Design review of the part built by this model. Coordinates are the model's own, in mm. A direction names the side the tool comes from. Round coordinates to 2 decimals unless told otherwise and drop trailing zeros. Order: outer loops, then holes, each group sorted by start corner. A loop starts at its lowest first (then second) coordinate and runs counter-clockwise, first axis right, second up. Notation, with made-up numbers: (70, -25.75) - (116, -25.75) arc R21 cw to (116, 13.25) - close; hole circle Ø6 at (-10, -35.75). An arc over 180 degrees is marked (long way). Write item = value, one per line.
from build123d import *

# Parameters (mm, degrees)
SKETCH_1_R          = 5
SKETCH_1_R_2        = 2.5
EXTRUDE_1_DEPTH     = 10
EXTRUDE_1_2_DEPTH   = 10
EXTRUDE_2_DEPTH     = 6
CUT_EXTRUDE_1_DEPTH = 4
SKETCH_5_R          = 2.5
EXTRUDE_3_DEPTH     = 2
CUT_EXTRUDE_2_DEPTH = 4


with BuildPart() as part:
    # Sketch 1 → Extrude 1 (new body)
    with BuildSketch(Plane.XY):
        with Locations((-11.277859903, 1.201925786)):
            Circle(SKETCH_1_R)
        with Locations((-11.277859903, 1.201925786)):
            Circle(SKETCH_1_R_2, mode=Mode.SUBTRACT)
    extrude(amount=EXTRUDE_1_DEPTH)



with BuildPart() as body_2:
    # Sketch 1 → Extrude 1 2 (new body)
    with BuildSketch(Plane.XY):
        with Locations((-37.440810807, -24.961025118)):
            Circle(SKETCH_1_R)
        with Locations((-37.440810807, -24.961025118)):
            Circle(SKETCH_1_R_2, mode=Mode.SUBTRACT)
    extrude(amount=EXTRUDE_1_2_DEPTH)


with BuildPart() as part_1:
    add(part.part)

    add(body_2.part)  # Extrude 2 merges body 2
    # Sketch 3 → Extrude 2 (add)
    with BuildSketch(Plane(origin=(0, 0, 0), x_dir=(-1, 0, 0), z_dir=(0, 0, -1))):
        Polygon((11.277859903, 1.201925786), (14.813393809, 4.737459692), (40.976344713, -21.425491212), (33.905276901, -28.496559024), (7.742325997, -2.33360812), align=None)
    extrude(amount=-EXTRUDE_2_DEPTH)

    # Sketch 4 → Cut-Extrude 1 (cut)
    with BuildSketch(Plane.XY.offset(6)):
        Polygon((-13.045626856, 2.969692739), (-9.51009295, -0.565841167), (-35.673043854, -26.728792071), (-39.20857776, -23.193258165), align=None)
    extrude(amount=-CUT_EXTRUDE_1_DEPTH, mode=Mode.SUBTRACT)

    # Sketch 5 → Extrude 3 (add)
    with BuildSketch(Plane(origin=(0, 0, 0), x_dir=(-1, 0, 0), z_dir=(0, 0, -1))):
        with Locations(Location((11.277859903, 1.201925786, 0), (0, 0, 45))):
            Circle(SKETCH_5_R)
        with Locations(Location((37.440810807, -24.961025118, 0), (0, 0, 45))):
            Circle(SKETCH_5_R)
    extrude(amount=-EXTRUDE_3_DEPTH)

    # Sketch 4_2 → Cut-Extrude 2 (cut)
    with BuildSketch(Plane.XY.offset(6)):
        Polygon((-13.045626856, 2.969692739), (-9.51009295, -0.565841167), (-35.673043854, -26.728792071), (-39.20857776, -23.193258165), align=None)
    extrude(amount=CUT_EXTRUDE_2_DEPTH, mode=Mode.SUBTRACT)


solid = part_1.part
1) The part is to be moulded in two halves that separate along X. For faces 3 (the flat face through (-21.01, -15.6, 2.96)), 4 (the flat face through (-24, -12, 2)), 5 (the cylindrical face through (-41.104, -28.365, 6.041)), 6 (the flat face through (-27, -9, 6)), say which applies: released by +X, released by -X, zero draft, split by the parting line, or undercut.
Findings:
face_3 = released by +X
face_4 = undercut
face_5 = split by the parting line
face_6 = zero draft
2) We need section B-B on y = -26. Write out the cut boundary in (x, z).
Findings:
outline = (-42.33, 0) - (-31.41, 0) - (-31.41, 6) - (-32.55, 6) - (-32.55, 10) - (-34.94, 10) - (-34.94, 2) - (-39.71, 2) - (-39.71, 10) - (-42.33, 10) - close
3) We need section D-D on z = 8. Write out the cut boundary in (x, y), and give its area (3 significant figures).
Findings:
outline = (-39.21, -23.19) - (-36.15, -20.13) arc R5 ccw (long way) to (-32.61, -23.67) - (-35.67, -26.73) arc R2.5 cw to start; (-16.11, -0.09) - (-13.05, 2.97) arc R2.5 cw to (-9.51, -0.57) - (-12.57, -3.63) arc R5 ccw (long way) to start
area = 89.6 mm^2
4) We need section A-A on z = 2.75. Write out the cut boundary in (x, y), and give its area (3 significant figures).
Findings:
outline = (-40.98, -21.43) arc R5 ccw to (-33.91, -28.5) - (-7.74, -2.33) arc R5 ccw to (-14.81, 4.74) - close; hole (-39.21, -23.19) arc R2.5 ccw to (-35.67, -26.73) - (-9.51, -0.57) arc R2.5 ccw to (-13.05, 2.97) - close
area = 244 mm^2
5) For faces 1 (the flat face through (-27.71, -8.16, 2.96)), 2 (the cylindrical face through (-9.47, 2.93, 5.94)), list the 3-axis set-ups (+Z, -Z, +X, -X, +Y, -Y) from which the entire face can be reached by the end or side of a thin tool; tool diameter is ignored.
Findings:
face_1 = +Z, -Z, -X, +Y
face_2 = +Z
6) We need section C-C on x = -13.5. Write out the cut boundary in (y, z).
Findings:
outline = (-8.09, 0) - (5.68, 0) - (5.68, 10) - (2.52, 10) - (2.52, 2) - (-4.56, 2) - (-4.56, 6) - (-8.09, 6) - close
7) To check wall thickness, follow L1, parallel to Z at x = -30.5, y = -21; L2, parallel to Z at x = -15, y = -7; L3, parallel to X at y = -1.5, z = 2.5. State the ranges of each line that lie inside material, in increasing order. Write a range as from..to.
Findings:
L1 = 0..2
L2 = 0..6
L3 = -21.05..-17.52, -10.44..-7.07
8) Clearance check with flat-ended pins moving along their axes: pin 1 Ø6 at (y, z) = (-12, 7.5) entering from -X; pin 2 Ø21 at (x, y) = (-21.5, -11.5) entering from +Z; pin 3 Ø1.5 at (x, z) = (-11, 3) entering from +Y; pin 4 Ø1.5 at (x, z) = (-31, 2) entering from +Y. State where each tip first meets the part, or that it passes through.
Findings:
pin_1 = -34.15
pin_2 = 6
pin_3 = 6.2
pin_4 = -10.7
